Could you check a few things on this model? Use its own coordinates, in mm. A direction names the side the tool comes from. Give positions to 0.01 mm unless a question says otherwise; leave off trailing zeros. Loops run counter-clockwise (first coordinate to the right, second up) from the corner with the lowest first, then second, coordinate; pieces in that order, holes last. Notation, with made-up numbers: M 66,35.25 L 118,35.25 A26 ccw 118,65.25 Z; hole C -11,-3.5 d9. An arc over 180 degrees is marked long. Use CSV: the item, a comma, the result in double quotes.
```python
from build123d import *

# Parameters (mm, degrees)
F0_R     = 1.75
F1_DEPTH = 12
F2_DEPTH = 25
F4_DEPTH = 75
F6_DEPTH = 10
F8_DEPTH = 10


# Not quite as in the source:
# - a feature names something its author has since deleted; it is built from what else it names


with BuildPart() as f1:
    # F0 (on Top) → F1 (new body)
    with BuildSketch(Plane.XY):
        with BuildLine():
            ThreePointArc((2.5, -4.6165463282), (0, -5.25), (-2.5, -4.6165463282))
            Line((-2.5, -4.6165463282), (-2.5, -54))
            Line((-2.5, -54), (-2.4, -54))
            Line((-2.4, -54), (2.4, -54))
            Line((2.4, -54), (2.5, -54))
            Line((2.5, -54), (2.5, -4.6165463282))
        make_face()
        with BuildLine():
            Line((-2.5, -4), (-2.5, -4.6165463282))
            ThreePointArc((-2.5, -4.6165463282), (0, -5.25), (2.5, -4.6165463282))
            Line((2.5, -4.6165463282), (2.5, -4))
            Line((2.5, -4), (-2.5, -4))
        make_face()
        with BuildLine():
            ThreePointArc((2.5, -4.6165463282), (4.5104046382, -2.6867731575), (5.25, 0))
            ThreePointArc((5.25, 0), (-2.6867731575, 4.5104046382), (-2.5, -4.6165463282))
            Line((-2.5, -4.6165463282), (-2.5, -4))
            Line((-2.5, -4), (2.5, -4))
            Line((2.5, -4), (2.5, -4.6165463282))
        make_face()
        Circle(F0_R, mode=Mode.SUBTRACT)
    extrude(amount=F1_DEPTH)

    # F0 (on Top) → F2 (join)
    with BuildSketch(Plane.XY):
        with BuildLine():
            Line((2.4, -54), (-2.4, -54))
            ThreePointArc((-2.4, -54), (-3.5313708499, -54.4686291501), (-4, -55.6))
            Line((-4, -55.6), (-4, -60.4))
            ThreePointArc((-4, -60.4), (-3.5313708499, -61.5313708499), (-2.4, -62))
            Line((-2.4, -62), (2.4, -62))
            ThreePointArc((2.4, -62), (3.5313708499, -61.5313708499), (4, -60.4))
            Line((4, -60.4), (4, -55.6))
            ThreePointArc((4, -55.6), (3.5313708499, -54.4686291501), (2.4, -54))
        make_face()
    extrude(amount=F2_DEPTH)

    # F3 (on face) → F4 (join)
    with BuildSketch(Plane.XY.offset(25)):
        with BuildLine():
            Line((2.4, -54), (0, -54))
            Line((0, -54), (0, -62))
            Line((0, -62), (2.4, -62))
            ThreePointArc((2.4, -62), (3.5313708499, -61.5313708499), (4, -60.4))
            Line((4, -60.4), (4, -55.6))
            ThreePointArc((4, -55.6), (3.5313708499, -54.4686291501), (2.4, -54))
        make_face()
    extrude(amount=F4_DEPTH)

    # F5 (on face) → F6 (cut)
    with BuildSketch(Plane.XY.offset(25)):
        with BuildLine():
            Line((-4, -58), (0, -58))
            Line((0, -58), (0, -54))
            Line((0, -54), (-2.4, -54))
            ThreePointArc((-2.4, -54), (-3.5313708499, -54.4686291501), (-4, -55.6))
            Line((-4, -55.6), (-4, -58))
        make_face()
    extrude(amount=-F6_DEPTH, mode=Mode.SUBTRACT)

    # F7 (on face) → F8 (join)
    with BuildSketch(Plane.XY.offset(100)):
        with BuildLine():
            Line((0, -58), (4, -58))
            Line((4, -58), (4, -55.6))
            ThreePointArc((4, -55.6), (3.5313708499, -54.4686291501), (2.4, -54))
            Line((2.4, -54), (0, -54))
            Line((0, -54), (0, -58))
        make_face()
    extrude(amount=F8_DEPTH)


solid = f1.part
```
1. I'm going to push flat-ended pins straight in: pin 1 Ø2 at (x, y) = (2, -59.5) entering from +Z; pin 2 Ø4 at (y, z) = (-59.5, 57.5) entering from -X; pin 3 Ø6 at (x, y) = (-2.5, -3.5) entering from +Z; pin 4 Ø3 at (x, y) = (0, 0) entering from +Z (1 decimal). Where does each tip first touch, or does it pass through?
Outcome:
pin 1,"z = 100"
pin 2,"x = 0"
pin 3,"z = 12"
pin 4,"through"
2. If we mould it in two halves opening along Y, with no side actions, what happens to faces 5 (the face through (-2, -58, 20)), 6 (the face through (2, -56, 110)), 7 (the face through (2.5, -30, 6)), 8 (the face through (1, -62, 38))? For each: +Y half, -Y half, draft (parallel to the pull), parting line (faces both ways), or undercut.
Outcome:
face 5,"+Y half"
face 6,"draft"
face 7,"undercut"
face 8,"-Y half"
3. I want a section at C-C, the plane y = -13.5. List the corners of the cut face in (x, z) for me.
Outcome:
outline,"M -2.5,0 L 2.5,0 L 2.5,12 L -2.5,12 Z"
4. I want a section at A-A, the plane y = 0. List the corners of the cut face in (x, z) for me, then the cut area to 3 significant figures.
Outcome:
outline,"M -5.25,0 L -1.75,0 L -1.75,12 L -5.25,12 Z; M 1.75,0 L 5.25,0 L 5.25,12 L 1.75,12 Z"
area,"84.0 mm2"
5. I want a section at B-B, the plane z = 93.5. List the corners of the cut face in (x, y) for me.
Outcome:
outline,"M 0,-62 L 2.4,-62 A1.6 ccw 4,-60.4 L 4,-55.6 A1.6 ccw 2.4,-54 L 0,-54 Z"
6. Please list where these lines run through material, in increasing order: line 1 (Y direction, x = 0, z = 7.5); line 2 (Z direction, x = 0, y = -14.5); line 3 (Y direction, x = 0.5, z = 67.5).
Outcome:
line 1,"-62 to -1.75, 1.75 to 5.25"
line 2,"0 to 12"
line 3,"-62 to -54"
7. Which directions (+Z, -Z, +X, -X, +Y, -Y) give clear straight access to the entire face, cutting with the end or side of a thin tool? Please do faces 1 (the face through (-4, -58, 10)), 2 (the face through (-2, -60, 25)), 3 (the face through (0, -24, 12)), 4 (the face through (2, -58, 105)).
Outcome:
face 1,"+Z, -Z, -X, -Y"
face 2,"+Z, -X, +Y, -Y"
face 3,"+Z, +X, -X, +Y"
face 4,"+Z, +X, -X, -Y"
